The listing builds one solid part. Answer for the finished solid, in the listing's coordinates (mm). Face numbers are marked on the shaded views. A direction names the side the tool comes from. Give positions to 0.01 mm unless a question says otherwise; leave off trailing zeros. Order: outer loops, then holes, each group sorted by start corner. A loop starts at its lowest first (then second) coordinate and runs counter-clockwise, first axis right, second up. Notation, with made-up numbers: (-16, 42.5) - (21, 42.5) arc R30 cw to (21, 79.5) - close; hole circle Ø1 at (46, 32). An arc over 180 degrees is marked (long way). Answer as CSV lines item,"result". Start each with the question number.
1. Consider line 1 along Z through (x, y) = (0, 24.15); line 2 along Z through (x, y) = (13, 18); line 3 along Z through (x, y) = (-11, 5). Determine where each line is inside the solid, lowest interval first. Write a range as [from, to].
2. Section C-C on y = 19 is taken. Give the vertices of the cut face in (x, z), and give its area (3 significant figures).
3. Flat-ended cylindrical pins translate along their axes: pin 1 (3.5 mm diameter, centred on x = 18.5, y = 23, fed in from +Z); pin 2 (5.5 mm diameter, centred on y = 25, z = 18.5, fed in from +X); pin 3 (4 mm diameter, centred on y = 25, z = 15, fed in from -X); pin 4 (10 mm diameter, centred on y = 10.5, z = 12.5, fed in from -X). Find the tip coordinate at first contact, or state that the pin passes through.
4. Section A-A on z = 13.5 is taken. Give the vertices of the cut face in (x, y).
5. Which of the six approach directions +Z, -Z, +X, -X, +Y, -Y give full straight-line access (tool end or side, diameter ignored) to the marked faces 4 and 5?
6. Section D-D on z = 17 is taken. Give the vertices of the cut face in (x, y), and give its area (3 significant figures).
7. Section B-B on x = -7 is taken. Give the vertices of the cut face in (y, z).
8. Determine the mould class of the marked faces 1, 2 and 3 for opening direction Y: +Y half, -Y half, draft (parallel to the pull), parting line (faces both ways), or undercut.
from build123d import *

# Parameters (mm, degrees)
SKETCH_W        = 45
SKETCH_H        = 50
PAD_DEPTH       = 3
SKETCH001_W     = 23
SKETCH001_H     = 25
PAD001_DEPTH    = 7
SKETCH002_W     = 45
SKETCH002_H     = 8
PAD002_DEPTH    = 3
POCKET_DEPTH    = 3
POCKET001_DEPTH = 3.5
SKETCH005_R     = 2.5
POCKET002_DEPTH = 50.501
FILLET_R        = 2.5
FILLET001_R     = 2


with BuildPart() as part:
    # Sketch → Pad (new body)
    with BuildSketch(Plane.XY):
        Rectangle(SKETCH_W, SKETCH_H)
    extrude(amount=PAD_DEPTH)

    # Sketch001 (on DatumPlane) → Pad001 (join)
    with BuildSketch(Plane(origin=(0, 22, 0), x_dir=(-1, 0, 0), z_dir=(0, 1, 0))):
        with Locations((0, 12.5)):
            Rectangle(SKETCH001_W, SKETCH001_H)
    extrude(amount=PAD001_DEPTH)

    # Sketch002 (on Face5 of Pad001) → Pad002 (join)
    with BuildSketch(Plane.XY.offset(3)):
        with Locations((0, 21)):
            Rectangle(SKETCH002_W, SKETCH002_H)
    extrude(amount=PAD002_DEPTH)

    # Sketch003 (on Face14 of Pad002) → Pocket (cut)
    with BuildSketch(Plane.XY.offset(6)):
        Polygon((-22.5, 22), (22.5, 22), (22.5, 19.7), (22.5, 17), (17.5, 17), (17.5, 19.7), (-17.5, 19.7), (-17.5, 17), (-22.5, 17), (-22.5, 19.7), align=None)
    extrude(amount=-POCKET_DEPTH, mode=Mode.SUBTRACT)

    # Sketch004 (on Face27 of Pocket) → Pocket001 (cut)
    with BuildSketch(Plane(origin=(0, 29, 0), x_dir=(-1, 0, 0), z_dir=(0, 1, 0))):
        Polygon((3.65, 11.392672), (3.65, 15.607328), (0, 17.714657), (-3.65, 15.607328), (-3.65, 11.392672), (0, 9.285343), align=None)
    extrude(amount=-POCKET001_DEPTH, mode=Mode.SUBTRACT)

    # Sketch005 (on Face34 of Pocket001) → Pocket002 (cut, through all)
    with BuildSketch(Plane(origin=(0, 25.5, 0), x_dir=(-1, 0, 0), z_dir=(0, 1, 0))):
        with Locations((0, 13.5)):
            Circle(SKETCH005_R)
    extrude(amount=-POCKET002_DEPTH, mode=Mode.SUBTRACT)

    # Fillet
    fillet_edges = [part.edges().sort_by_distance(p)[0] for p in [
        (0, 17, 3),
    ]]
    fillet(fillet_edges, radius=FILLET_R)

    # Fillet001
    fillet001_edges = [part.edges().sort_by_distance(p)[0] for p in [
        (0, 29, 25),
        (11.5, 29, 12.5),
        (-11.5, 29, 12.5),
    ]]
    fillet(fillet001_edges, radius=FILLET001_R)


solid = part.part
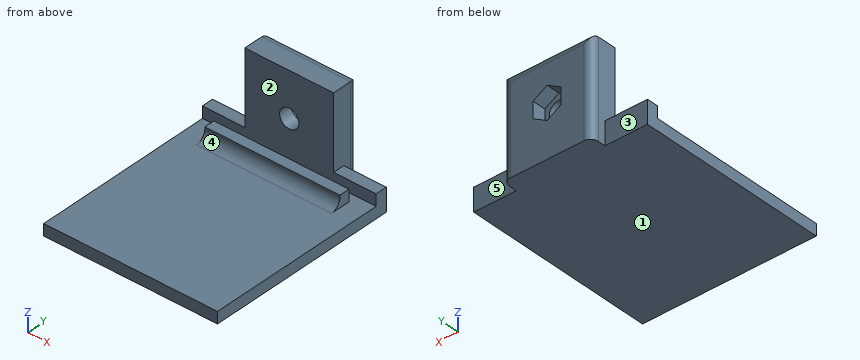
Checks:
1,line 1,"z = [0, 11], [16, 25]"
1,line 2,"z = [0, 6]"
1,line 3,"z = [0, 3]"
2,outline,"(-22.5, 0) - (22.5, 0) - (22.5, 3) - (17.5, 3) - (17.5, 6) - (-17.5, 6) - (-17.5, 3) - (-22.5, 3) - close"
2,area,"240 mm²"
3,pin 1,"stops at z = 6"
3,pin 2,"stops at x = 11.5"
3,pin 3,"stops at x = -11.5"
3,pin 4,"passes through"
4,outline,"(-11.5, 22) - (-2.5, 22) - (-2.5, 25.5) - (-3.65, 25.5) - (-3.65, 29) - (-9.5, 29) arc R2 ccw to (-11.5, 27) - close; (2.5, 22) - (11.5, 22) - (11.5, 27) arc R2 ccw to (9.5, 29) - (3.65, 29) - (3.65, 25.5) - (2.5, 25.5) - close"
5,face 4,"+Z, +X, -X, -Y"
5,face 5,"+Z, -Z, +X, +Y"
6,outline,"(-11.5, 22) - (11.5, 22) - (11.5, 27) arc R2 ccw to (9.5, 29) - (1.24, 29) - (1.24, 25.5) - (-1.24, 25.5) - (-1.24, 29) - (-9.5, 29) arc R2 ccw to (-11.5, 27) - close"
6,area,"151 mm²"
7,outline,"(-25, 0) - (29, 0) - (29, 23) arc R2 ccw to (27, 25) - (22, 25) - (22, 3) - (19.7, 3) - (19.7, 6) - (17, 6) - (17, 5.5) arc R2.5 cw to (14.5, 3) - (-25, 3) - close"
8,face 1,"draft"
8,face 2,"undercut"
8,face 3,"+Y half"
